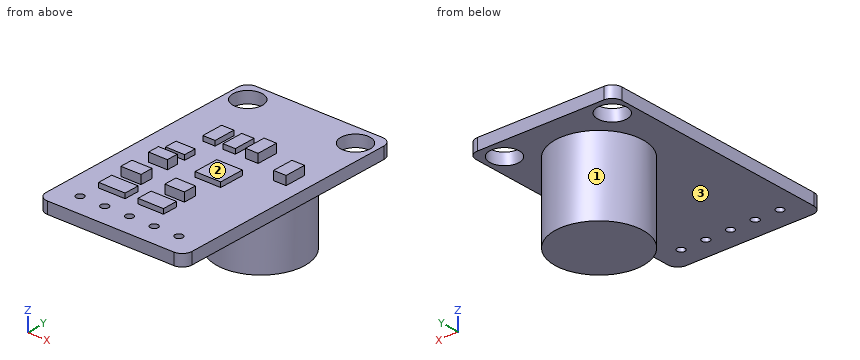
from build123d import *

# Parameters (mm, degrees)
BOSS_EXTRUDE1_DEPTH                  = 1.2
SKETCH2_R                            = 4.5
BOSS_EXTRUDE2_DEPTH                  = 8
F_3_0MM_DOWEL_HOLE1_D                = 3
F_3_0MM_DOWEL_HOLE1_DEPTH            = 2
F_3_0MM_DOWEL_HOLE1_TIP              = 0.901290929
F_97_0_03149606_DIAMETER_HOLE1_D     = 0.799999924
F_97_0_03149606_DIAMETER_HOLE1_DEPTH = 2
F_97_0_03149606_DIAMETER_HOLE1_TIP   = 0.240344225
SKETCH17_W                           = 2.632057762
SKETCH17_H                           = 2.598740575
BOSS_EXTRUDE5_DEPTH                  = 0.5
SKETCH18_W                           = 2.719328156
SKETCH18_H                           = 1.56361369
SKETCH18_W_2                         = 2.61735335
BOSS_EXTRUDE6_DEPTH                  = 0.5
SKETCH19_W                           = 2.073487719
SKETCH19_H                           = 1.325672476
SKETCH19_W_2                         = 2.005504515
BOSS_EXTRUDE7_DEPTH                  = 0.9
SKETCH20_W                           = 1.971512913
SKETCH20_H                           = 1.257689272
SKETCH20_W_2                         = 1.257689272
SKETCH20_H_2                         = 2.243445728
SKETCH20_W_3                         = 1.257689273
BOSS_EXTRUDE8_DEPTH                  = 0.5
SKETCH21_W                           = 1.937521311
SKETCH21_H                           = 1.189706068
SKETCH21_W_2                         = 1.291680874
SKETCH21_H_2                         = 2.209454126
BOSS_EXTRUDE9_DEPTH                  = 0.9


with BuildPart() as part:
    # Sketch1 → Boss-Extrude1 (new body)
    with BuildSketch(Plane.XY):
        with BuildLine():
            Line((1, 0), (14, 0))
            ThreePointArc((14, 0), (14.707106781, -0.292893219), (15, -1))
            Line((15, -1), (15, -24))
            ThreePointArc((15, -24), (14.707106781, -24.707106781), (14, -25))
            Line((14, -25), (1, -25))
            ThreePointArc((1, -25), (0.292893219, -24.707106781), (0, -24))
            Line((0, -24), (0, -1))
            ThreePointArc((0, -1), (0.292893219, -0.292893219), (1, 0))
        make_face()
    extrude(amount=BOSS_EXTRUDE1_DEPTH)

    # Sketch2 → Boss-Extrude2 (add)
    with BuildSketch(Plane.XY):
        with Locations((7.5, -7)):
            Circle(SKETCH2_R)
    extrude(amount=-BOSS_EXTRUDE2_DEPTH)

    # Ø3.0mm Dowel Hole1
    with Locations(Plane(origin=(0, 0, 0), x_dir=(-1, 0, 0), z_dir=(0, 0, -1))):
        with Locations((-13.006639516, -2.081574002), (-1.92537728, -2.081574002)):
            Hole(F_3_0MM_DOWEL_HOLE1_D / 2, depth=F_3_0MM_DOWEL_HOLE1_DEPTH)
            with Locations((0, 0, -(F_3_0MM_DOWEL_HOLE1_DEPTH + F_3_0MM_DOWEL_HOLE1_TIP / 2))):  # 118° drill point
                Cone(0, F_3_0MM_DOWEL_HOLE1_D / 2, F_3_0MM_DOWEL_HOLE1_TIP, mode=Mode.SUBTRACT)

    # #97 (0.03149606) Diameter Hole1
    with Locations(Plane(origin=(0, 0, 0), x_dir=(-1, 0, 0), z_dir=(0, 0, -1))):
        with Locations((-7.5, -22.748467988), (-10.04, -22.748467988), (-12.58, -22.748467988), (-4.96, -22.748467988), (-2.42, -22.748467988)):
            Hole(F_97_0_03149606_DIAMETER_HOLE1_D / 2, depth=F_97_0_03149606_DIAMETER_HOLE1_DEPTH)
            with Locations((0, 0, -(F_97_0_03149606_DIAMETER_HOLE1_DEPTH + F_97_0_03149606_DIAMETER_HOLE1_TIP / 2))):  # 118° drill point
                Cone(0, F_97_0_03149606_DIAMETER_HOLE1_D / 2, F_97_0_03149606_DIAMETER_HOLE1_TIP, mode=Mode.SUBTRACT)

    # Sketch17 → Boss-Extrude5 (add)
    with BuildSketch(Plane.XY.offset(1.2)):
        with Locations((8.499275401, -13.218640589)):
            Rectangle(SKETCH17_W, SKETCH17_H)
    extrude(amount=BOSS_EXTRUDE5_DEPTH)

    # Sketch18 → Boss-Extrude6 (add)
    with BuildSketch(Plane.XY.offset(1.2)):
        with Locations((3.998864999, -19.99514823)):
            Rectangle(SKETCH18_W, SKETCH18_H)
        with Locations((7.992878228, -19.99514823)):
            Rectangle(SKETCH18_W_2, SKETCH18_H)
    extrude(amount=BOSS_EXTRUDE6_DEPTH)

    # Sketch19 → Boss-Extrude7 (add)
    with BuildSketch(Plane.XY.offset(1.2)):
        with Locations((3.743927985, -17.530757089)):
            Rectangle(SKETCH19_W, SKETCH19_H)
        with Locations((8.230819441, -17.530757089)):
            Rectangle(SKETCH19_W_2, SKETCH19_H)
    extrude(amount=BOSS_EXTRUDE7_DEPTH)

    # Sketch20 → Boss-Extrude8 (add)
    with BuildSketch(Plane.XY.offset(1.2)):
        with Locations((3.760923786, -12.296050388)):
            Rectangle(SKETCH20_W, SKETCH20_H)
        with Locations((4.389768422, -8.471995169)):
            Rectangle(SKETCH20_W_2, SKETCH20_H_2)
        with Locations((6.463256141, -8.471995169)):
            Rectangle(SKETCH20_W_3, SKETCH20_H_2)
    extrude(amount=BOSS_EXTRUDE8_DEPTH)

    # Sketch21 → Boss-Extrude9 (add)
    with BuildSketch(Plane.XY.offset(1.2)):
        with Locations((3.777919587, -14.403529709)):
            Rectangle(SKETCH21_W, SKETCH21_H)
        with Locations((8.791680874, -8.48899097)):
            Rectangle(SKETCH21_W_2, SKETCH21_H_2)
        with Locations((12.836681506, -9.848655048)):
            Rectangle(SKETCH21_W_2, SKETCH21_H_2)
    extrude(amount=BOSS_EXTRUDE9_DEPTH)


solid = part.part
Work out the finished part from the listing and answer in its coordinate system (mm). Face numbers are marked on the shaded views. Round coordinates to 2 decimals unless told otherwise and drop trailing zeros. Write each loop counter-clockwise with the first axis right and the second up, starting at its lowest first coordinate (ties: lowest second). Pieces come first, ordered by that corner, then holes. Notation, with made-up numbers: M 63.5,37 L 115.5,37 A26 ccw 115.5,56 Z; hole C -19,-35.75 d8. An arc over 180 degrees is marked long. Use a Markdown table: item, result.
1) The part is cut by section C-C on z = 0.5. Give the vertices of the cut face in (x, y), plus the area to 3 significant figures.
Taken from the geometry:
| item | result |
|---|---|
| outline | M 0,-24 A1 ccw 1,-25 L 14,-25 A1 ccw 15,-24 L 15,-1 A1 ccw 14,0 L 1,0 A1 ccw 0,-1 Z; hole C 1.93,-2.08 d3; hole C 2.42,-22.75 d0.8; hole C 4.96,-22.75 d0.8; hole C 7.5,-22.75 d0.8; hole C 10.04,-22.75 d0.8; hole C 13.01,-2.08 d3; hole C 12.58,-22.75 d0.8 |
| area | 357 mm2 |
2) Consider line 1 (Y direction, x = 4.96, z = 0.85); line 2 (Z direction, x = 3.25, y = -7.5); line 3 (Y direction, x = 13.5, z = 0.75). Determine where each line is inside the solid, lowest interval first. Write a range as [from, to].
Taken from the geometry:
| item | result |
|---|---|
| line 1 | y = [-25, -23.15], [-22.35, 0] |
| line 2 | z = [-8, 1.2] |
| line 3 | y = [-25, -3.5], [-0.67, 0] |
3) Determine the mould class of the marked faces 1, 2 and 3 for opening direction Z: pulls with the +Z half, pulls with the -Z half, needs draft (parallel to the pull), parting line crosses it, or undercut.
Taken from the geometry:
| item | result |
|---|---|
| face 1 | needs draft |
| face 2 | pulls with the +Z half |
| face 3 | pulls with the -Z half |
4) Flat-ended cylindrical pins translate along their axes: pin 1 (1 mm diameter, centred on y = -17.5, z = 2, fed in from +X); pin 2 (7.5 mm diameter, centred on x = 9, y = -18.5, fed in from -Z); pin 3 (3 mm diameter, centred on y = -7, z = -3, fed in from -X); pin 4 (4 mm diameter, centred on y = -15.5, z = -3, fed in from -X). Find the tip coordinate at first contact, or state that the pin passes through.
Taken from the geometry:
| item | result |
|---|---|
| pin 1 | stops at x = 9.23 |
| pin 2 | stops at z = 0 |
| pin 3 | stops at x = 3 |
| pin 4 | passes through |
5) The part is cut by section D-D on z = -4.75. Give the vertices of the cut face in (x, y), plus the area to 3 significant figures.
Taken from the geometry:
| item | result |
|---|---|
| outline | C 7.5,-7 d9 |
| area | 63.6 mm2 |
6) The part is cut by section B-B on x = 12.58. Give the vertices of the cut face in (y, z).
Taken from the geometry:
| item | result |
|---|---|
| outline | M -25,0 L -23.15,0 L -23.15,1.2 L -25,1.2 Z; M -22.35,0 L -3.52,0 L -3.52,1.2 L -8.74,1.2 L -8.74,2.1 L -10.95,2.1 L -10.95,1.2 L -22.35,1.2 Z; M -0.64,0 L 0,0 L 0,1.2 L -0.64,1.2 Z |
7) The part is cut by section A-A on y = -7. Give the vertices of the cut face in (x, z).
Taken from the geometry:
| item | result |
|---|---|
| outline | M 0,0 L 3,0 L 3,-8 L 12,-8 L 12,0 L 15,0 L 15,1.2 L 0,1.2 Z |
